```python
from build123d import *

# Parameters (mm, degrees)
SWEEP1_PROFILE_R   = 26.67
CUT_EXTRUDE1_START = -45.72
SKETCH2_R          = 26.67
SKETCH2_R_2        = 3.81
CUT_EXTRUDE1_DEPTH = 45.72
SHELL1_START       = -150.978
SHELL1_OUTLINE_R   = 23.368
SHELL1_DEPTH       = 192.278
SHELL1_START_2     = -197.46
SHELL1_2_OUTLINE_R = 1.27
SHELL1_2_DEPTH     = 46.482
SKETCH3_R          = 1.27
CUT_EXTRUDE2_DEPTH = 252.433520836


# Read off the part's stored shape, not the designer's step: Shell1
with BuildPart() as part:
    # Sweep1: sweep along a path in Sketch1
    with BuildLine(Plane(origin=(0, 0, 0), x_dir=(1, 0, 0), z_dir=(0, 1, 0))) as sweep1_path:
        Line((-200, 47.5), (41.3, 47.5))
    # Sweep1 profile (on start of the path) → Sweep1 (sweep)
    with BuildSketch(Plane(origin=(-200, 0, -47.5), x_dir=(0, 0, 1), z_dir=(1, 0, 0))):
        Circle(SWEEP1_PROFILE_R)
    sweep(path=sweep1_path.line)

    # Sketch2 → Cut-Extrude1 (cut)
    with BuildSketch(Plane.ZY.offset(200).offset(CUT_EXTRUDE1_START)):
        with Locations(Location((-47.5, 0, 0), (0, 0, 180))):
            Circle(SKETCH2_R)
        with Locations((-47.5, 0)):
            Circle(SKETCH2_R_2, mode=Mode.SUBTRACT)
    extrude(amount=CUT_EXTRUDE1_DEPTH, mode=Mode.SUBTRACT)

    # Shell1 outline → Shell1 (cut)
    with BuildSketch(Plane.YZ.offset(SHELL1_START)):
        with Locations((0, -47.5)):
            Circle(SHELL1_OUTLINE_R)
    extrude(amount=SHELL1_DEPTH, mode=Mode.SUBTRACT)

    # Shell1 2 outline → Shell1 2 (cut)
    with BuildSketch(Plane.YZ.offset(SHELL1_START_2)):
        with Locations((0, -47.5)):
            Circle(SHELL1_2_OUTLINE_R)
    extrude(amount=SHELL1_2_DEPTH, mode=Mode.SUBTRACT)

    # Sketch3 → Cut-Extrude2 (cut, through all)
    with BuildSketch(Plane(origin=(-197.46, 0, 0), x_dir=(0, 0, -1), z_dir=(1, 0, 0))):
        with Locations(Location((47.5, 0, 0), (0, 0, 180))):
            Circle(SKETCH3_R)
    extrude(amount=-CUT_EXTRUDE2_DEPTH, mode=Mode.SUBTRACT)


solid = part.part
```
Geometry: final body of the model. Coordinates: model frame, mm. A direction names the side the tool comes from. Coordinates: 2 decimals unless noted, no trailing zeros. Order: outer loops, then holes, each group sorted by start corner. A loop starts at its lowest first (then second) coordinate and runs counter-clockwise, first axis right, second up. Notation, with made-up numbers: (80.25, 51.25) -> (97.25, 51.25) arc R32 ccw to (97.25, 77.25) -> close; hole circle Ø4 at (63.5, -32). An arc over 180 degrees is marked (long way). Write item = value, one per line.
(1) Cut plane C-C on z = -41.5. Return loops of the section in (x, y).
Solved:
outline = (-154.28, -25.99) -> (41.3, -25.99) -> (41.3, -22.58) -> (-150.98, -22.58) -> (-150.98, 22.58) -> (41.3, 22.58) -> (41.3, 25.99) -> (-154.28, 25.99) -> close
(2) Cut plane A-A on y = -12. Return loops of the section in (x, z), plus the area to 3 significant figures.
Solved:
outline = (-154.28, -71.32) -> (41.3, -71.32) -> (41.3, -67.55) -> (-150.98, -67.55) -> (-150.98, -27.45) -> (41.3, -27.45) -> (41.3, -23.68) -> (-154.28, -23.68) -> close
area = 1,610 mm²
(3) Cut plane B-B on x = -28.5. Return loops of the section in (y, z), plus the area to 3 significant figures.
Solved:
outline = circle Ø53.34 at (0, -47.5); hole circle Ø46.74 at (0, -47.5)
area = 519 mm²
(4) Pull-direction query (Z, two-part tool) for faces 1 (the cylindrical face through (-176.82, -1.46, -43.98)), 2 (the flat face through (-200, 0, -46)), 3 (the cylindrical face through (-56.18, -5.07, -70.31)); classes: pulls with the +Z half, pulls with the -Z half, needs draft (parallel to the pull), parting line crosses it, or undercut.
Solved:
face_1 = parting line crosses it
face_2 = needs draft
face_3 = undercut
(5) Pin query (flat end, axial travel): pin 1 Ø12 at (x, y) = (-119, 17.5) entering from +Z; pin 2 Ø5 at (x, z) = (-94, -58) entering from +Y; pin 3 Ø8 at (y, z) = (-12, -55.5) entering from -X. Return the tip coordinate at first contact, or that it passes through.
Solved:
pin_1 = -23.44
pin_2 = 25.44
pin_3 = -154.28
(6) Line query: line 1 (Y direction, x = -168.5, z = -47.5); line 2 (Y direction, x = -73, z = -48.5); line 3 (Z direction, x = -12.5, y = 0). Output: solid intervals per line, ascending.
Solved:
line_1 = -3.81 to -1.27, 1.27 to 3.81
line_2 = -26.65 to -23.35, 23.35 to 26.65
line_3 = -74.17 to -70.87, -24.13 to -20.83
(7) Access query for faces 4 (the flat face through (-150.978, 0, -52)), 5 (the flat face through (41.3, 24, -48)). Directions: +Z, -Z, +X, -X, +Y, -Y. A direction counts if a zero-diameter tool reaches every point of the face in a straight line with its end or side. Return the directions, or none.
Solved:
face_4 = +X
face_5 = +Z, -Z, +X, +Y, -Y
